from build123d import *

# Parameters (mm, degrees)
BASE_EXTRUDE_DEPTH      = 40.132
BASE_EXTRUDE_DEPTH_BACK = 40.132
SKETCH5_R               = 27.94
BOSS_EXTRUDE1_DEPTH     = 457.2


with BuildPart() as part:
    # Sketch4 → Base-Extrude (new, two sides: drawn at the far end of the back side and taken through both)
    with BuildSketch(Plane.XY.offset(-BASE_EXTRUDE_DEPTH_BACK)):
        with BuildLine():
            Line((0.868, 60), (168, 60))
            ThreePointArc((168, 60), (228, 0), (168, -60))
            Line((168, -60), (0.868, -60))
            Line((0.868, -60), (0.868, 60))
        make_face()
    extrude(amount=BASE_EXTRUDE_DEPTH + BASE_EXTRUDE_DEPTH_BACK)

    # Sketch5 → Boss-Extrude1 (add)
    with BuildSketch(Plane.ZY.offset(-0.868)):
        with Locations(Location((0, 0, 0), (0, 0, 180))):
            Circle(SKETCH5_R)
    extrude(amount=BOSS_EXTRUDE1_DEPTH)


solid = part.part
Design review of the part built by this model. Coordinates are the model's own, in mm. Round coordinates to 2 decimals unless told otherwise and drop trailing zeros. Write each loop counter-clockwise with the first axis right and the second up, starting at its lowest first coordinate (ties: lowest second). Pieces come first, ordered by that corner, then holes. Notation, with made-up numbers: (45.25, 49) -> (86.25, 49) arc R15 cw to (86.25, 54) -> close; hole circle Ø11 at (22, 65). An arc over 180 degrees is marked (long way). One line per item, written item: value. Start each with the question number.
Q1. Add section A-A (y = 0). Give the boundary of the cut face in (x, z), then the cut area to 3 significant figures.
Q2. The part is to be moulded in two halves that separate along X. For faces 1 (the face through (-224.53, -27.7, 3.64)), 2 (the face through (227.985, 1.319, -0.562)), 3 (the face through (0.868, -28, 8)), say which applies: pulls with the +X half, pulls with the -X half, needs draft (parallel to the pull), parting line crosses it, or undercut.
Q3. To check wall thickness, follow probe 1 along X at (y, z) = (-4, -28.5); probe 2 along Y at (x, z) = (-303, 1.5); probe 3 along Y at (x, z) = (-131, -10.5). State the ranges of each line that lie inside material, in increasing order.
Q4. Add section C-C (x = -336.5). Give the boundary of the cut face in (y, z).
Q5. Add section D-D (y = -35). Give the boundary of the cut face in (x, z).
Q6. Insertion check: P1, Ø3, axis at x = -312.5, y = -17.5, coming from the +Z side; P2, Ø8, axis at y = -47.5, z = -4, coming from the +X side; P3, Ø10, axis at x = -140, z = -18.5, coming from the -Y side. Each pin has a flat end and moves straight along its axis. Give the tip position at first contact, or say it passes through.
Q7. Add section B-B (z = 0). Give the boundary of the cut face in (x, y), then the cut area to 3 significant figures.
Response:
1. outline: (-456.33, -27.94) -> (0.87, -27.94) -> (0.87, -40.13) -> (228, -40.13) -> (228, 40.13) -> (0.87, 40.13) -> (0.87, 27.94) -> (-456.33, 27.94) -> close
1. area: 43,800 mm^2
2. face 1: needs draft
2. face 2: pulls with the +X half
2. face 3: pulls with the -X half
3. probe 1: x = 0.87 to 227.87
3. probe 2: y = -27.9 to 27.9
3. probe 3: y = -25.89 to 25.89
4. outline: circle Ø55.88 at (0, 0)
5. outline: (0.87, -40.13) -> (216.73, -40.13) -> (216.73, 40.13) -> (0.87, 40.13) -> close
6. P1: stops at z = 22.91
6. P2: stops at x = 209.32
6. P3: stops at y = -24.46
7. outline: (-456.33, -27.94) -> (0.87, -27.94) -> (0.87, -60) -> (168, -60) arc R60 ccw to (168, 60) -> (0.87, 60) -> (0.87, 27.94) -> (-456.33, 27.94) -> close
7. area: 51,300 mm^2
